```python
from build123d import *

# Parameters (mm, degrees)
SKETCH_1_R               = 57.8
EXTRUDE_1_DEPTH          = 3
SKETCH_2_R               = 1.75
CUT_EXTRUDE_1_DEPTH      = 82.796576945
PATTERN_CIRCULAR_1_COUNT = 12
SKETCH_3_R               = 2.1
CUT_EXTRUDE_2_DEPTH      = 82.796576945
PATTERN_CIRCULAR_2_COUNT = 6
SKETCH_4_R               = 1.49
CUT_EXTRUDE_3_DEPTH      = 82.796576945
PATTERN_CIRCULAR_3_COUNT = 6
SKETCH_5_R               = 2.7
SKETCH_5_R_2             = 11.5
CUT_EXTRUDE_4_DEPTH      = 82.796576945
PATTERN_CIRCULAR_4_COUNT = 6
CHAMFER_1_SIZE           = 2.5


with BuildPart() as part:
    # 草图1 → 凸台-拉伸1 (new body)
    with BuildSketch(Plane(origin=(0, 0, 0), x_dir=(1, 0, 0), z_dir=(0, 1, 0))):
        with Locations(Location((0, 0, 0), (0, 0, 270))):
            Circle(SKETCH_1_R)
    extrude(amount=EXTRUDE_1_DEPTH)

    # 草图2 → 切除-拉伸1 (cut, symmetric)
    with BuildSketch(Plane.XZ):
        with Locations(Location((0, 54, 0), (0, 0, 270))):
            Circle(SKETCH_2_R)
    cut_extrude_1 = extrude(amount=CUT_EXTRUDE_1_DEPTH, both=True, mode=Mode.SUBTRACT)

    # 阵列(圆周)1: 切除-拉伸1 ×12 about axis
    pattern_circular_1_axis = Axis((0, 0, 0), (0, 1, 0))
    for i in range(1, PATTERN_CIRCULAR_1_COUNT):
        add(cut_extrude_1.rotate(pattern_circular_1_axis, i * 360 / PATTERN_CIRCULAR_1_COUNT), mode=Mode.SUBTRACT)

    # 草图3 → 切除-拉伸2 (cut, symmetric)
    with BuildSketch(Plane.XZ):
        with Locations(Location((0, 30, 0), (0, 0, 270))):
            Circle(SKETCH_3_R)
    cut_extrude_2 = extrude(amount=CUT_EXTRUDE_2_DEPTH, both=True, mode=Mode.SUBTRACT)

    # 阵列(圆周)2: 切除-拉伸2 ×6 about axis
    pattern_circular_2_axis = Axis((0, 0, 0), (0, 1, 0))
    for i in range(1, PATTERN_CIRCULAR_2_COUNT):
        add(cut_extrude_2.rotate(pattern_circular_2_axis, i * 360 / PATTERN_CIRCULAR_2_COUNT), mode=Mode.SUBTRACT)

    # 草图4 → 切除-拉伸3 (cut, symmetric)
    with BuildSketch(Plane.XZ):
        with Locations(Location((31, 0, 0), (0, 0, 270))):
            Circle(SKETCH_4_R)
    cut_extrude_3 = extrude(amount=CUT_EXTRUDE_3_DEPTH, both=True, mode=Mode.SUBTRACT)

    # 阵列(圆周)3: 切除-拉伸3 ×6 about axis
    pattern_circular_3_axis = Axis((0, 0, 0), (0, 1, 0))
    for i in range(1, PATTERN_CIRCULAR_3_COUNT):
        add(cut_extrude_3.rotate(pattern_circular_3_axis, i * 360 / PATTERN_CIRCULAR_3_COUNT), mode=Mode.SUBTRACT)

    # 草图5 → 切除-拉伸4 (cut, symmetric)
    with BuildSketch(Plane(origin=(0, 3, 0), x_dir=(1, 0, 0), z_dir=(0, 1, 0))):
        with Locations(Location((17.5, 0, 0), (0, 0, 270))):
            Circle(SKETCH_5_R)
        with Locations(Location((0, 0, 0), (0, 0, 270))):
            Circle(SKETCH_5_R_2)
    cut_extrude_4 = extrude(amount=CUT_EXTRUDE_4_DEPTH, both=True, mode=Mode.SUBTRACT)

    # 阵列(圆周)4: 切除-拉伸4 ×6 about axis
    pattern_circular_4_axis = Axis((0, 0, 0), (0, 1, 0))
    for i in range(1, PATTERN_CIRCULAR_4_COUNT):
        add(cut_extrude_4.rotate(pattern_circular_4_axis, i * 360 / PATTERN_CIRCULAR_4_COUNT), mode=Mode.SUBTRACT)

    # 倒角1
    chamfer_1_edges = [part.edges().sort_by_distance(p)[0] for p in [
        (17.5, 3, -2.7),
        (-11.08826859, 3, -13.805444566),
        (6.41173141, 3, -16.505444566),
        (-6.41173141, 3, 16.505444566),
        (-17.5, 3, 2.7),
        (11.08826859, 3, 13.805444566),
    ]]
    chamfer(chamfer_1_edges, length=CHAMFER_1_SIZE)


solid = part.part
```
Geometry check sheet. Reference: the model listing, model coordinates, mm. Coordinates: 2 decimals unless noted, no trailing zeros. Write each loop counter-clockwise with the first axis right and the second up, starting at its lowest first coordinate (ties: lowest second). Pieces come first, ordered by that corner, then holes. Notation, with made-up numbers: M 57.25,-35.75 L 92.25,-35.75 A21 ccw 92.25,-21.75 Z; hole C 23.5,34.25 d3. An arc over 180 degrees is marked long. One line per item, written item: value. Start each with the question number.
(1) Sectioned sample at C-C, the plane x = -31. Enter the section's corners in (y, z).
(2) Release check for a two-part mould opening along X. For faces 1 (the face through (48.74, 1.48, 31.07)), 2 (the face through (9.78, 0.25, 12.66)) record: released by +X, released by -X, zero draft, split by the parting line, or undercut.
(3) Sectioned sample at D-D, the plane z = -22.5. Enter the section's corners in (x, y), and give its area (3 significant figures).
(4) Depth check by flat-ended pin: pin 1 (5 mm diameter, centred on x = -8.75, z = 15.16, fed in from -Y). Enter the tip coordinate at first touch or a pass-through.
(5) Sectioned sample at A-A, the plane x = -54. Enter the section's corners in (y, z).
(6) Scan lines: line 1 along X through (y, z) = (1.3, -2.5); line 2 along X through (y, z) = (0.25, -15); line 3 along Z through (x, y) = (-1.5, 1.1). Record each from-to range of solid material in increasing order. Write a range as [from, to].
(7) Sectioned sample at B-B, the plane y = 1.9. State how many separate pieces and enclosed holes the cut face has, and give its area (3 significant figures).
Filled sheet:
1. outline: M 0,-48.78 L 3,-48.78 L 3,-1.49 L 0,-1.49 Z; M 0,1.49 L 3,1.49 L 3,48.78 L 0,48.78 Z
2. face 1: split by the parting line
2. face 2: undercut
3. outline: M -53.24,0 L 53.24,0 L 53.24,3 L -53.24,3 Z
3. area: 319 mm²
4. pin 1: through
5. outline: M 0,-20.61 L 3,-20.61 L 3,-1.75 L 0,-1.75 Z; M 0,1.75 L 3,1.75 L 3,20.61 L 0,20.61 Z
6. line 1: [-57.75, -19.95], [-15.05, -11.22], [11.22, 15.05], [19.95, 57.75]
6. line 2: [-55.82, -28.08], [-23.88, -11.45], [-6.05, 6.05], [11.45, 23.88], [28.08, 55.82]
6. line 3: [-57.78, -54.9], [-53.1, -31.47], [-28.53, -11.4], [11.4, 28.53], [31.47, 53.1], [54.9, 57.78]
7. separate pieces: 1
7. enclosed holes: 31
7. area: 9,520 mm²
